Could you check a few things on this drawing? It's one solid part, dimensions in mm from its lowest x, y, z. A direction names the side the tool comes from. Give positions to 0.01 mm unless a question says otherwise; leave off trailing zeros. Order: outer loops, then holes, each group sorted by start corner. A loop starts at its lowest first (then second) coordinate and runs counter-clockwise, first axis right, second up. Notation, with made-up numbers: (65.5, -28.75) - (75.5, -28.75) arc R12 ccw to (75.5, -24.75) - close; hole circle Ø11 at (74, 34). An arc over 180 degrees is marked (long way). Return JSON: item names as keys, results as strings.
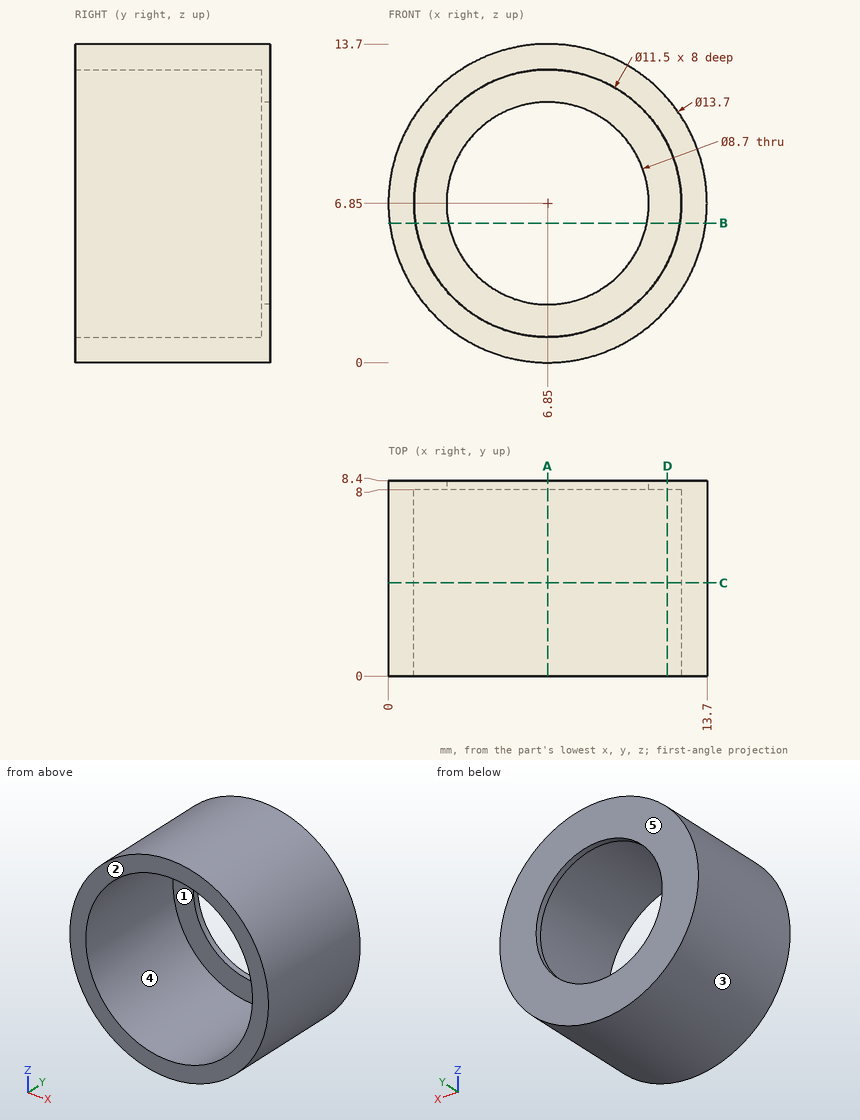
1. Thinking about a two-plate mould opening in Z: for the marked faces 1, 2 and 3, which applies, +Z half, -Z half, draft (parallel to the pull), parting line (faces both ways), or undercut?
Checks:
{"face 1": "undercut", "face 2": "draft", "face 3": "parting line"}
2. On a 3-axis mill with a long thin cutter (end or side, diameter ignored), from which of +Z, -Z, +X, -X, +Y, -Y can I reach the whole of each face in a straight line? I mean the marked faces 4 and 5. Say none if no direction works.
Checks:
{"face 4": "-Y", "face 5": "+Z, -Z, +X, -X, +Y"}
3. Suppose I cut it at C-C (y = 4). List the corners of the cut face in (x, z) for me.
Checks:
{"outline": "circle Ø13.7 at (6.85, 6.85); hole circle Ø11.5 at (6.85, 6.85)"}
4. For pin 1 Ø2 at (x, z) = (7.5, 9) entering from -Y, with a flat end and sliding along its axis, tell me the tip position at first contact or that it passes through.
Checks:
{"pin 1": "through"}
5. If I drill on L1, parallel to Z at x = 6.85, y = 3.75; L2, parallel to Z at x = 6.85, y = 8.1; L3, parallel to Y at x = 5, z = 12, over which ranges is the centre line in solid material (lowest first)? Write a range as [from, to].
Checks:
{"L1": "[0, 1.1], [12.6, 13.7]", "L2": "[0, 2.5], [11.2, 13.7]", "L3": "[8, 8.4]"}
6. Suppose I cut it at A-A (x = 6.85). List the corners of the cut face in (y, z) for me, plus the area to 3 significant figures.
Checks:
{"outline": "(0, 0) - (8.4, 0) - (8.4, 2.5) - (8, 2.5) - (8, 1.1) - (0, 1.1) - close; (0, 12.6) - (8, 12.6) - (8, 11.2) - (8.4, 11.2) - (8.4, 13.7) - (0, 13.7) - close", "area": "19.6 mm^2"}
7. Suppose I cut it at D-D (x = 12). List the corners of the cut face in (y, z) for me, plus the area to 3 significant figures.
Checks:
{"outline": "(0, 2.33) - (8.4, 2.33) - (8.4, 11.37) - (0, 11.37) - (0, 9.41) - (8, 9.41) - (8, 4.29) - (0, 4.29) - close", "area": "35.0 mm^2"}
8. Suppose I cut it at B-B (z = 6). List the corners of the cut face in (x, y) for me, plus the area to 3 significant figures.
Checks:
{"outline": "(0.05, 0) - (1.16, 0) - (1.16, 8) - (2.58, 8) - (2.58, 8.4) - (0.05, 8.4) - close; (11.12, 8) - (12.54, 8) - (12.54, 0) - (13.65, 0) - (13.65, 8.4) - (11.12, 8.4) - close", "area": "19.8 mm^2"}
